Autodesk Inventor part; units mm, degrees
ref_plane "YZ Plane" through (0, 0, 0) normal (1, 0, 0) x (0, 1, 0)
ref_plane "XZ Plane" through (0, 0, 0) normal (0, 1, 0) x (-1, 0, 0)
ref_plane "XY Plane" through (0, 0, 0) normal (0, 0, 1) x (1, 0, 0)
sketch "Sketch1" plane through (0, 0, 0) normal (1, 0, 0) x (0, 1, 0)
  line L0 (-6.35, 6.35) -> (6.35, 6.35)
  line L1 (6.35, 6.35) -> (6.35, -6.35)
  line L2 (6.35, -6.35) -> (-6.35, -6.35)
  line L3 (-6.35, -6.35) -> (-6.35, 6.35)
  line L4 (-6.35, 6.35) -> (6.35, -6.35) construction
  line L5 (6.35, 6.35) -> (-6.35, -6.35) construction
  point P0 (0, 0)
  dimension "d0" = 12.7
  dimension "d1" = 12.7
extrude "Extrusion1" add sketch "Sketch1" along normal mid plane 100
chamfer "Chamfer1" distance 6.35 angle 45 1 edges at (0, -6.35, -6.35)
fillet "Fillet1" radius 12.7 1 edges at (0, 6.35, 6.35)
sketch "Sketch2" plane through (50, 0, -6.35) normal (0, 0, -1) x (-1, 0, 0)
  line L0 (100, 0) -> (0, 0)
  line L1 (100, 6.35) -> (100, 0)
  line L2 (0, 6.35) -> (100, 6.35)
  line L3 (0, 0) -> (0, 6.35)
  circle A0 centre (100, 0) radius 1.5875
  line L4 (0, -6.35) -> (100, -6.35)
  line L5 (100, 0) -> (0, 0)
  line L6 (98.4125, 0) -> (98.4125, -6.35)
  line L7 (101.5875, 0) -> (101.5875, -6.35)
  line L8 (101.5875, -6.35) -> (98.4125, -6.35)
  point P0 (50, 0)
  dimension "d8" = 3.175
revolve "Revolution1" cut sketch "Sketch2" angle 360 about axis through (50, -6.35, -6.35) along (-1, 0, 0) contours L1 A0 L0 | L0 A0 L1 | A0 L7 L8 L4 L6
mirror "Mirror1" about plane through (0, 0, 0) normal (1, 0, 0) of "Revolution1"
equation "\"d0\" = facingThickness"
equation "\"d1\" = facingThickness"
equation "\"d2\" = depth"
equation "\"d4\" = 0.5 * facingThickness"
equation "\"d7\" = facingThickness"
equation "\"d8\" = 0.25 * facingThickness"
equation "\"mppcMountThickness\" = 6.35"
equation "\"depth\" = 100"
equation "\"facingThickness\" = 12.7"
equation "\"facingGasketThickness\" = 1.5875"
properties part number "sideMoulding" material "Wood (Cherry)"
Here's how the part is built. I have some questions about the finished solid (model axes, mm). A direction names the side the tool comes from. Coordinates: 2 decimals unless noted, no trailing zeros. Loops run counter-clockwise (first coordinate to the right, second up) from the corner with the lowest first, then second, coordinate; pieces in that order, holes last.
1. For P1, Ø5, axis at y = -4.5, z = -3.5, coming from the -X side; P2, Ø1.5, axis at x = -6.5, y = -3.5, coming from the -Z side; P3, Ø4, axis at x = -35.5, y = -5, coming from the +Z side; P4, Ø5, axis at y = -2.5, z = -3, coming from the +X side, each with a flat end and sliding along its axis, tell me the tip position at first contact or that it passes through.
2. Imagine slicing it at B-B, the plane y = 4. Please give me the cut outline in (x, z).
3. I need wall thicknesses on L1, parallel to Y at x = 31.5, z = 0.5; L2, parallel to Y at x = 41.5, z = -5; L3, parallel to Z at x = 4, y = 2.75. Which ranges of each line are inside material? Lowest first, please.
4. For faces 1 (the flat face through (-48.412, -3, -3)), 2 (the flat face through (48.412, -3, -3)), 3 (the flat face through (-1, -6.35, 3)), which set-ups out of +Z, -Z, +X, -X, +Y, -Y let a thin tool reach every point of the face, with its end or its side?
Taken from the geometry:
1. P1: stops at x = -48.41
1. P2: stops at z = -3.6
1. P3: stops at z = 6.35
1. P4: stops at x = 49.03
2. outline: (-50, -6.35) - (50, -6.35) - (50, 1.01) - (-50, 1.01) - close
3. L1: y = -6.35 to 4.34
3. L2: y = -1.35 to 6.28
3. L3: z = -6.35 to 2.51
4. face 1: -Z, -X, -Y
4. face 2: -Z, +X, -Y
4. face 3: +Z, -Z, +X, -X, -Y
